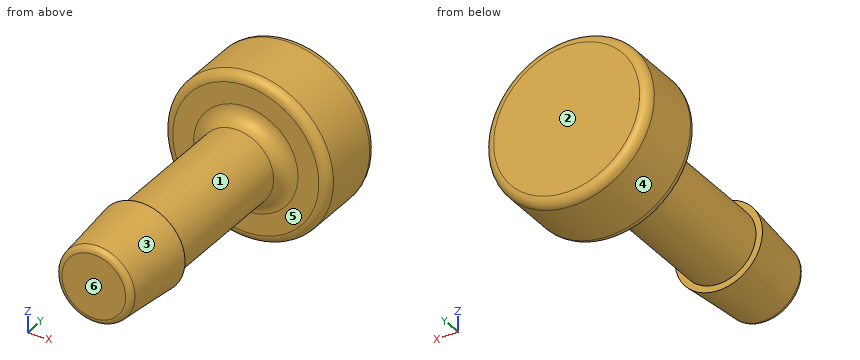
from build123d import *

# Parameters (mm, degrees)
FILLET_R    = 0.4
FILLET001_R = 1
FILLET002_R = 0.6


with BuildPart() as part:
    # Sketch → Revolution (revolve)
    with BuildSketch(Plane.YZ):
        Polygon((-10.5, 2.5), (-5.5, 2.935), (-5.5, 2.5), (5.5, 2.5), (5.5, 5.5), (10.5, 5.5), (10.5, 0), (-10.5, 0), align=None)
    revolve(axis=Axis((0, 0, 0), (0, 1, 0)))

    # Fillet
    fillet_edges = [part.edges().sort_by_distance(p)[0] for p in [
        (0, -10.5, -2.5),
    ]]
    fillet(fillet_edges, radius=FILLET_R)

    # Fillet001
    fillet001_edges = [part.edges().sort_by_distance(p)[0] for p in [
        (0, 5.5, -2.5),
    ]]
    fillet(fillet001_edges, radius=FILLET001_R)

    # Fillet002
    fillet002_edges = [part.edges().sort_by_distance(p)[0] for p in [
        (0, 5.5, -5.5),
        (0, 10.5, -5.5),
    ]]
    fillet(fillet002_edges, radius=FILLET002_R)


solid = part.part
Design review of the part built by this model. Coordinates are the model's own, in mm. Face numbers are marked on the shaded views. A direction names the side the tool comes from. Coordinates: 2 decimals unless noted, no trailing zeros. Loops run counter-clockwise (first coordinate to the right, second up) from the corner with the lowest first, then second, coordinate; pieces in that order, holes last. Notation, with made-up numbers: (78, 80) -> (102, 80) arc R12 ccw to (102, 96) -> close; hole circle Ø4 at (43.5, -16). An arc over 180 degrees is marked (long way). Use a Markdown table: item, result. Add a question column.
Item 1: The part is to be moulded in two halves that separate along Y. For the marked faces 1, 2, 3 and 4, say which applies: +Y half, -Y half, draft (parallel to the pull), parting line (faces both ways), or undercut.
Item 2: Clearance check with flat-ended pins moving along their axes: P1, Ø5, axis at y = 7.5, z = 3, coming from the +X side; P2, Ø1, axis at x = -2, z = -4, coming from the -Y side; P3, Ø4, axis at x = -3, y = 2.5, coming from the -Z side. State where each tip first meets the part, or that it passes through.
Item 3: We need section B-B, the plane z = 0. Write out the cut boundary in (x, y) (3 decimals), and give its area (3 significant figures).
Item 4: We need section C-C, the plane y = 7. Write out the cut boundary in (x, z), and give its area (3 significant figures).
Item 5: We need section D-D, the plane y = 0.5. Write out the cut boundary in (x, z).
Item 6: Wall thickness on L1, parallel to Y at x = 2, z = -3.5; L2, parallel to X at y = 4.5, z = -1.5; L3, parallel to Z at x = -0.5, y = 5: over which ranges is each line inside the solid? List them lowest first. Write a range as from..to.
Item 7: We need section A-A, the plane x = 0. Write out the cut boundary in (y, z) (3 decimals), and give its area (3 significant figures).
Item 8: Machinability: for the marked faces 5 and 6, which of the approach directions +Z, -Z, +X, -X, +Y, -Y give a long, thin tool a straight path to every point of the face, cutting with its end or side? Answer none if there is none.
Numbers:
| question | item | result |
|---|---|---|
| 1 | face 1 | undercut |
| 1 | face 2 | +Y half |
| 1 | face 3 | -Y half |
| 1 | face 4 | draft |
| 2 | P1 | stops at x = 5.48 |
| 2 | P2 | stops at y = 5.5 |
| 2 | P3 | stops at z = -2.29 |
| 3 | outline | (-5.5, 6.1) arc R0.6 ccw to (-4.9, 5.5) -> (-3.5, 5.5) arc R1 cw to (-2.5, 4.5) -> (-2.5, -5.5) -> (-2.935, -5.5) -> (-2.532, -10.135) arc R0.4 ccw to (-2.133, -10.5) -> (2.133, -10.5) arc R0.4 ccw to (2.532, -10.135) -> (2.935, -5.5) -> (2.5, -5.5) -> (2.5, 4.5) arc R1 cw to (3.5, 5.5) -> (4.9, 5.5) arc R0.6 ccw to (5.5, 6.1) -> (5.5, 9.9) arc R0.6 ccw to (4.9, 10.5) -> (-4.9, 10.5) arc R0.6 ccw to (-5.5, 9.9) -> close |
| 3 | area | 137 mm^2 |
| 4 | outline | circle Ø11 at (0, 0) |
| 4 | area | 95.0 mm^2 |
| 5 | outline | circle Ø5 at (0, 0) |
| 6 | L1 | y = 5.5..10.5 |
| 6 | L2 | x = -2..2 |
| 6 | L3 | z = -2.59..2.59 |
| 7 | outline | (-10.5, -2.133) arc R0.4 ccw to (-10.135, -2.532) -> (-5.5, -2.935) -> (-5.5, -2.5) -> (4.5, -2.5) arc R1 cw to (5.5, -3.5) -> (5.5, -4.9) arc R0.6 ccw to (6.1, -5.5) -> (9.9, -5.5) arc R0.6 ccw to (10.5, -4.9) -> (10.5, 4.9) arc R0.6 ccw to (9.9, 5.5) -> (6.1, 5.5) arc R0.6 ccw to (5.5, 4.9) -> (5.5, 3.5) arc R1 cw to (4.5, 2.5) -> (-5.5, 2.5) -> (-5.5, 2.935) -> (-10.135, 2.532) arc R0.4 ccw to (-10.5, 2.133) -> close |
| 7 | area | 137 mm^2 |
| 8 | face 5 | -Y |
| 8 | face 6 | +Z, -Z, +X, -X, -Y |
